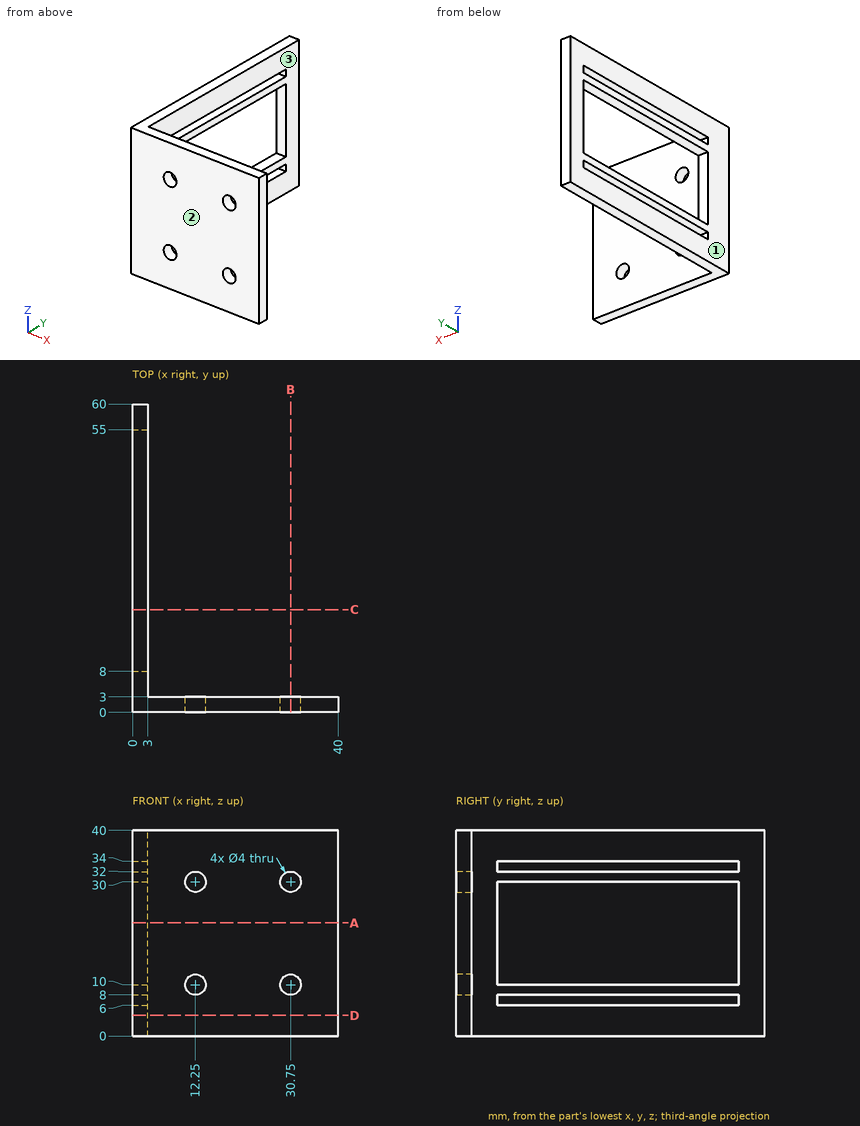
Input: dimensioned drawing with shaded views. Units: mm. Origin: part minimum x, y, z. Round coordinates to 2 decimals unless told otherwise and drop trailing zeros. Loops run counter-clockwise (first coordinate to the right, second up) from the corner with the lowest first, then second, coordinate; pieces in that order, holes last. Notation, with made-up numbers: (53.5, -28.5) -> (97.5, -28.5) arc R26 cw to (97.5, 3.5) -> close; hole circle Ø5 at (-28.5, 26.25). An arc over 180 degrees is marked (long way). One line per item, written item: value.
(1) Section D-D (z = 4). Return the cut outline in (x, y).
Geometry check:
outline: (0, 0) -> (40, 0) -> (40, 3) -> (3, 3) -> (3, 60) -> (0, 60) -> close
(2) Section A-A (z = 22). Return the cut outline in (x, y), plus the area to 3 significant figures.
Geometry check:
outline: (0, 0) -> (40, 0) -> (40, 3) -> (3, 3) -> (3, 8) -> (0, 8) -> close; (0, 55) -> (3, 55) -> (3, 60) -> (0, 60) -> close
area: 150 mm2
(3) Material intervals for line 1 (X direction, y = 2, z = 10); line 2 (Z direction, x = 12, y = 1); line 3 (X direction, y = 32.5, z = 2.5), sorted ascending. Write a range as [from, to].
Geometry check:
line 1: [0, 10.25], [14.25, 28.75], [32.75, 40]
line 2: [0, 8.02], [11.98, 28.02], [31.98, 40]
line 3: [0, 3]
(4) Section C-C (y = 20). Return the cut outline in (x, z).
Geometry check:
outline: (0, 0) -> (3, 0) -> (3, 6) -> (0, 6) -> close; (0, 8) -> (3, 8) -> (3, 10) -> (0, 10) -> close; (0, 30) -> (3, 30) -> (3, 32) -> (0, 32) -> close; (0, 34) -> (3, 34) -> (3, 40) -> (0, 40) -> close
(5) Section B-B (x = 30.75). Return the cut outline in (y, z).
Geometry check:
outline: (0, 0) -> (3, 0) -> (3, 8) -> (0, 8) -> close; (0, 12) -> (3, 12) -> (3, 28) -> (0, 28) -> close; (0, 32) -> (3, 32) -> (3, 40) -> (0, 40) -> close
(6) Pin query (flat end, axial travel): pin 1 (1.5 mm diameter, centred on x = 31, z = 24.5, fed in from +Y). Return the tip coordinate at first contact, or that it passes through.
Geometry check:
pin 1: y = 3
(7) Mould query, pull axis X, two halves, no side actions, for the marked faces 1, 2 and 3. Classes: pulls with the +X half, pulls with the -X half, needs draft (parallel to the pull), parting line crosses it, or undercut.
Geometry check:
face 1: pulls with the -X half
face 2: needs draft
face 3: pulls with the +X half
